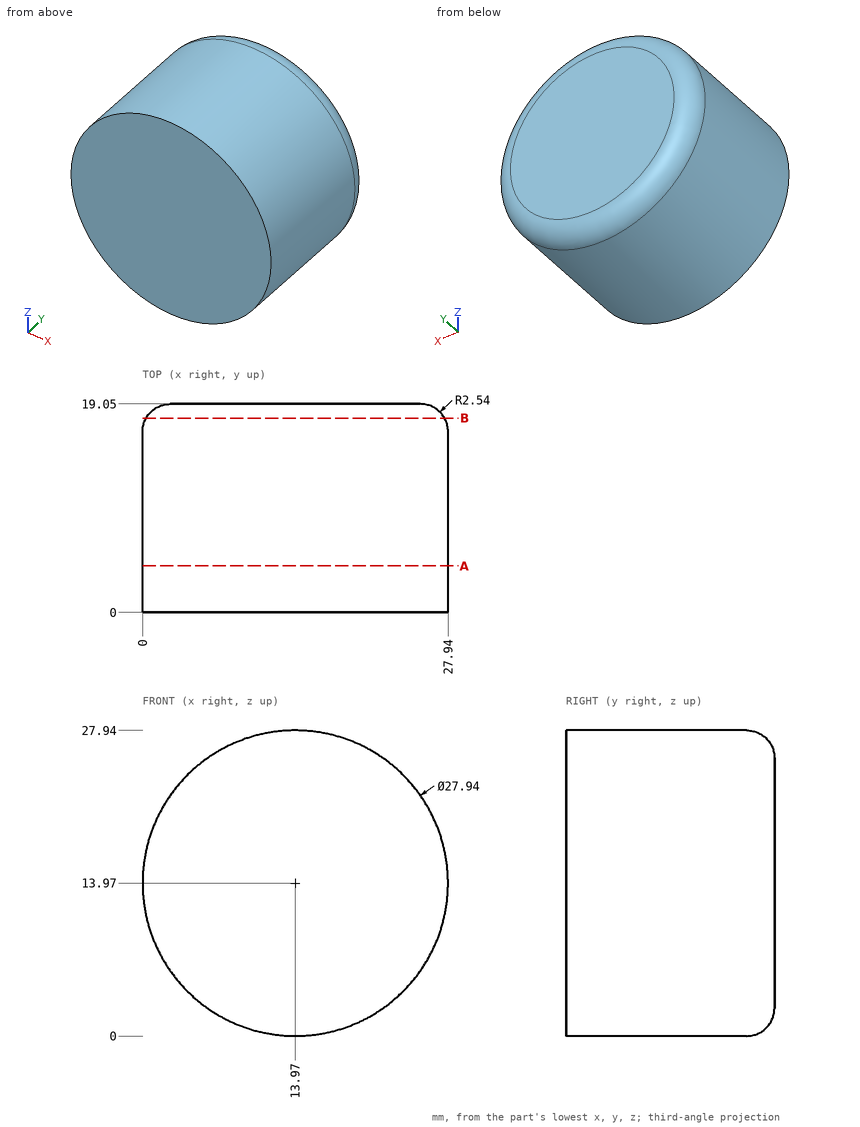
Design review of the part shown in the three views and the two pictorial views. Dimensions are in mm from the part's minimum x, y and z. Give positions to 0.01 mm unless a question says otherwise; leave off trailing zeros. Loops run counter-clockwise (first coordinate to the right, second up) from the corner with the lowest first, then second, coordinate; pieces in that order, holes last. Notation, with made-up numbers: (-39, -4.75) -> (-33, -4.75) arc R17 ccw to (-33, 3.25) -> close; hole circle Ø2 at (13.5, 34). An arc over 180 degrees is marked (long way). One line per question, with ' | ' between items.
1) Insertion check: pin 1 Ø5 at (y, z) = (11, 23.5) entering from +X; pin 2 Ø1.5 at (x, y) = (10.5, 6) entering from -Z; pin 3 Ø6 at (y, z) = (5, 5) entering from +X. Each pin has a flat end and moves straight along its axis. Give the tip position at first contact, or say it passes through.
Resolved:
pin 1: stops at x = 26.04 | pin 2: stops at z = 0.27 | pin 3: stops at x = 26.6
2) We need section A-A (y = 4.25). Write out the cut boundary in (x, z).
Resolved:
outline: circle Ø27.94 at (13.97, 13.97)
3) We need section B-B (y = 17.75). Write out the cut boundary in (x, z), plus the area to 3 significant figures.
Resolved:
outline: circle Ø27.29 at (13.97, 13.97) | area: 585 mm2
4) To check wall thickness, follow probe 1 along Z at (x, y) = (20.25, 1); probe 2 along X at (y, z) = (5.25, 22.5); probe 3 along X at (y, z) = (9.25, 19.5). State the ranges of each line that lie inside material, in increasing order.
Resolved:
probe 1: z = 1.49 to 26.45 | probe 2: x = 2.91 to 25.03 | probe 3: x = 1.14 to 26.8
